Verification items for the finished model (mm, model axes). Face numbers are marked on the shaded views. Round coordinates to 2 decimals unless told otherwise and drop trailing zeros. Order: outer loops, then holes, each group sorted by start corner. A loop starts at its lowest first (then second) coordinate and runs counter-clockwise, first axis right, second up.
Autodesk Inventor part; units mm, degrees
ref_plane "YZ Plane" through (0, 0, 0) normal (1, 0, 0) x (0, 1, 0)
ref_plane "XZ Plane" through (0, 0, 0) normal (0, 1, 0) x (-1, 0, 0)
ref_plane "XY Plane" through (0, 0, 0) normal (0, 0, 1) x (1, 0, 0)
sketch "Sketch1" plane through (0, 0, 0) normal (0, 1, 0) x (-1, 0, 0)
  arc A0 (20, 0) -> (-20, 0) centre (0, 0) ccw
  line L0 (20, 0) -> (20, -24)
  line L1 (20, -24) -> (-20, -24)
  line L2 (-20, -24) -> (-20, 0)
  dimension "d0" = 40
  dimension "d1" = 44
extrude "Extrusion1" add sketch "Sketch1" along normal blind 2.5
sketch "Sketch2" plane through (0, 2.5, 0) normal (0, 1, 0) x (1, 0, 0)
  arc A0 (-20, 0) -> (20, 0) centre (0, 0) ccw
  circle A1 centre (0, 0) radius 18
  circle A2 centre (0, 0) radius 16
  arc A3 (-15.7218, 2.9708) -> (-15.9996, 0.1135) centre (-15.4272, 1.5) ccw
  arc A4 (15.9996, 0.1135) -> (15.7218, 2.9708) centre (15.4272, 1.5) ccw
  line L0 (-15.9249, 1.5484) -> (-16.9202, 1.6452) construction
  line L1 (16.9202, 1.6452) -> (15.9249, 1.5484) construction
  dimension "d4" = 36
  dimension "d7" = 2
  dimension "d8" = 3
  dimension "d9" = 1
  dimension "d10" = 1.5
extrude "Extrusion2" add sketch "Sketch2" along normal blind 2.5
sketch "Sketch3" plane through (0, 2.5, 0) normal (0, 1, 0) x (1, 0, 0)
  arc A0 (-15.9996, 0.1135) -> (15.9996, 0.1135) centre (0, 0) ccw
  circle A1 centre (0, 0) radius 3.125
  dimension "d13" = 6.25
extrude "Extrusion3" cut sketch "Sketch3" against normal through all
sketch "Sketch4" plane through (0, 2.5, 0) normal (0, 1, 0) x (1, 0, 0)
  circle A0 centre (0, 0) radius 3.125
  circle A1 centre (-8, 0) radius 0.625
  dimension "d16" = 1.25
  dimension "d18" = 8
extrude "Extrusion4" add sketch "Sketch4" along normal blind 1 contours A1
sketch "Sketch5" plane through (0, 2.5, 0) normal (0, 1, 0) x (1, 0, 0)
  circle A0 centre (0, 0) radius 3.125
  circle A1 centre (7.7782, 7.7782) radius 1.435
  circle A2 centre (-7.7782, -7.7782) radius 1.435
  line L0 (7.7782, 7.7782) -> (-7.7782, -7.7782) construction
  line L1 (20, 24) -> (-20, 24) construction
  dimension "d21" = 2.87
  dimension "d23" = 22
  dimension "d24" = 45
extrude "Extrusion5" cut sketch "Sketch5" against normal through all contours A1 | A2
properties part number "WhitePumpBase"
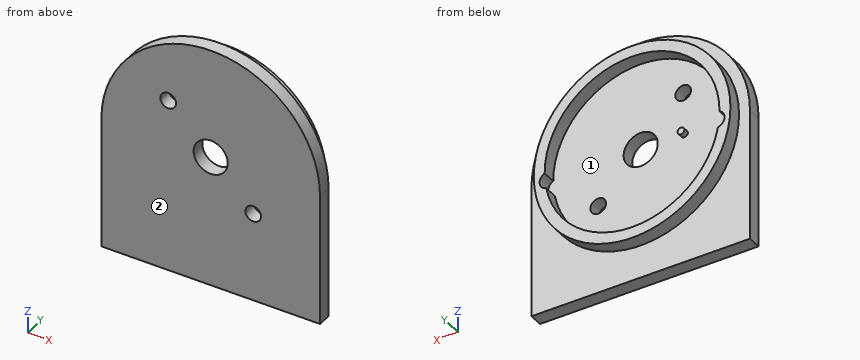
1) Sectioned sample at C-C on y = 1.5. Record the cut outline in (x, z) (3 decimals).
2) Sectioned sample at A-A on x = 0. Record the cut outline in (y, z) (3 decimals), then the cut area to 3 significant figures.
3) Sectioned sample at B-B on z = 2. Record the cut outline in (x, y).
4) Go/stop test with flat-tipped pins: pin 1 Ø2 at (x, z) = (-6.5, 10.5) entering from +Y; pin 2 Ø1.7 at (x, z) = (7.78, -7.78) entering from +Y; pin 3 Ø9.5 at (x, z) = (-7, 0) entering from +Y; pin 4 Ø1.5 at (y, z) = (3, 11.5) entering from -X. Record where each tip stops, or that it passes through.
5) Draft check along X on the marked faces 1 and 2. Enter one of: released by +X, released by -X, zero draft, split by the parting line, or undercut.
6) Scan lines: probe 1 along X at (y, z) = (2.05, 0) (3 decimals); probe 2 along Z at (x, y) = (0, 0.9) (3 decimals); probe 3 along Y at (x, z) = (-15, -22). Record each from-to range of solid material in increasing order.
7) Sectioned sample at D-D on x = -8. Record the cut outline in (y, z) (3 decimals), then the cut area to 3 significant figures.
Returned:
1. outline: (-20, -24) - (20, -24) - (20, 0) arc R20 ccw to (-20, 0) - close; hole circle Ø2.87 at (-7.778, 7.778); hole circle Ø6.25 at (0, 0); hole circle Ø2.87 at (7.778, -7.778)
2. outline: (0, -24) - (2.5, -24) - (2.5, -18) - (5, -18) - (5, -16) - (2.5, -16) - (2.5, -3.125) - (0, -3.125) - close; (0, 3.125) - (2.5, 3.125) - (2.5, 16) - (5, 16) - (5, 18) - (2.5, 18) - (2.5, 20) - (0, 20) - close
2. area: 104 mm2
3. outline: (-19.9, 0) - (-2.4, 0) - (-2.4, 2.5) - (-15.87, 2.5) - (-15.87, 5) - (-17.89, 5) - (-17.89, 2.5) - (-19.9, 2.5) - close; (2.4, 0) - (19.9, 0) - (19.9, 2.5) - (17.89, 2.5) - (17.89, 5) - (15.87, 5) - (15.87, 2.5) - (2.4, 2.5) - close
4. pin 1: stops at y = 2.5
4. pin 2: passes through
4. pin 3: stops at y = 3.5
4. pin 4: stops at x = -16.74
5. face 1: undercut
5. face 2: zero draft
6. probe 1: x = -20 to -3.125, 3.125 to 20
6. probe 2: z = -24 to -3.125, 3.125 to 20
6. probe 3: y = 0 to 2.5
7. outline: (0, -24) - (2.5, -24) - (2.5, -16.125) - (5, -16.125) - (5, -13.856) - (2.5, -13.856) - (2.5, -0.625) - (3.5, -0.625) - (3.5, 0.625) - (2.5, 0.625) - (2.5, 6.36) - (0, 6.36) - close; (0, 9.196) - (2.5, 9.196) - (2.5, 13.856) - (5, 13.856) - (5, 16.125) - (2.5, 16.125) - (2.5, 18.33) - (0, 18.33) - close
7. area: 111 mm2
